from build123d import *

# Parameters (mm, degrees)
EXTRUDE_1_DEPTH        = 195
CUT_EXTRUDE_1_DEPTH    = 10
PATTERN_LINEAR_1_COUNT = 50
PATTERN_LINEAR_1_PITCH = 20


with BuildPart() as part:
    # 草图1 → 凸台-拉伸1 (new, symmetric)
    with BuildSketch(Plane.XY):
        with BuildLine():
            Line((0, 19.218912653), (1, 19.218912653))
            Line((1, 19.218912653), (1, 16.218912653))
            ThreePointArc((1, 16.218912653), (0.414213562, 14.80469909), (-1, 14.218912653))
            Line((-1, 14.218912653), (-4.5, 14.218912653))
            ThreePointArc((-4.5, 14.218912653), (-5.207106781, 13.926019434), (-5.5, 13.218912653))
            Line((-5.5, 13.218912653), (-5.5, -9.781087347))
            ThreePointArc((-5.5, -9.781087347), (-5.207106781, -10.488194128), (-4.5, -10.781087347))
            Line((-4.5, -10.781087347), (-1, -10.781087347))
            ThreePointArc((-1, -10.781087347), (0.414213562, -11.366873785), (1, -12.781087347))
            Line((1, -12.781087347), (1, -15.781087347))
            Line((1, -15.781087347), (0, -15.781087347))
            Line((0, -15.781087347), (0, -12.781087347))
            ThreePointArc((0, -12.781087347), (-0.292893219, -12.073980566), (-1, -11.781087347))
            Line((-1, -11.781087347), (-4.5, -11.781087347))
            ThreePointArc((-4.5, -11.781087347), (-5.914213562, -11.19530091), (-6.5, -9.781087347))
            Line((-6.5, -9.781087347), (-6.5, 13.218912653))
            ThreePointArc((-6.5, 13.218912653), (-5.914213562, 14.633126215), (-4.5, 15.218912653))
            Line((-4.5, 15.218912653), (-1, 15.218912653))
            ThreePointArc((-1, 15.218912653), (-0.292893219, 15.511805872), (0, 16.218912653))
            Line((0, 16.218912653), (0, 19.218912653))
        make_face()
    extrude(amount=EXTRUDE_1_DEPTH, both=True)

    # 草图2 → 切除-拉伸1 (cut)
    with BuildSketch(Plane(origin=(-5.5, 0, 0), x_dir=(0, 0, -1), z_dir=(1, 0, 0))):
        with BuildLine():
            Line((-183.75, 3.718912653), (-176.25, 3.718912653))
            ThreePointArc((-176.25, 3.718912653), (-174.25, 1.718912653), (-176.25, -0.281087347))
            Line((-176.25, -0.281087347), (-183.75, -0.281087347))
            ThreePointArc((-183.75, -0.281087347), (-185.75, 1.718912653), (-183.75, 3.718912653))
        make_face()
    cut_extrude_1 = extrude(amount=-CUT_EXTRUDE_1_DEPTH, mode=Mode.SUBTRACT)

    # 阵列(线性)1: 切除-拉伸1 ×50
    with Locations(*[(0, 0, -i * PATTERN_LINEAR_1_PITCH) for i in range(1, PATTERN_LINEAR_1_COUNT)]):
        add(cut_extrude_1, mode=Mode.SUBTRACT)


solid = part.part
Input: part model. Units: mm. Frame: model coordinates. Give positions to 0.01 mm unless a question says otherwise; leave off trailing zeros. Order: outer loops, then holes, each group sorted by start corner. A loop starts at its lowest first (then second) coordinate and runs counter-clockwise, first axis right, second up. Notation, with made-up numbers: M 40.25,64.5 L 97.25,64.5 A27 cw 97.25,83.5 Z; hole C -34,-20 d2. An arc over 180 degrees is marked long. Answer as a JSON object with one key per item and string values.
1. Cut plane A-A, the plane x = -3. Output: boundary loops of the cut face in (y, z), and give its area (3 significant figures).
Result sheet:
{"outline": "M -11.78,-195 L -10.78,-195 L -10.78,195 L -11.78,195 Z; M 14.22,-195 L 15.22,-195 L 15.22,195 L 14.22,195 Z", "area": "780 mm²"}
2. Pull-direction query (Y, two-part tool) for faces 1 (the flat face through (-6, -8, -195)), 2 (the flat face through (-5.5, -1, 3)); classes: +Y half, -Y half, draft (parallel to the pull), parting line (faces both ways), or undercut.
Result sheet:
{"face 1": "draft", "face 2": "undercut"}
3. Cut plane B-B, the plane z = 111. Output: boundary loops of the cut face in (x, y), and give its area (3 significant figures).
Result sheet:
{"outline": "M -6.5,-9.78 A2 ccw -4.5,-11.78 L -1,-11.78 A1 cw 0,-12.78 L 0,-15.78 L 1,-15.78 L 1,-12.78 A2 ccw -1,-10.78 L -4.5,-10.78 A1 cw -5.5,-9.78 L -5.5,13.22 A1 cw -4.5,14.22 L -1,14.22 A2 ccw 1,16.22 L 1,19.22 L 0,19.22 L 0,16.22 A1 cw -1,15.22 L -4.5,15.22 A2 ccw -6.5,13.22 Z", "area": "45.4 mm²"}
4. First-contact query: P1, Ø1.5, axis at y = 3, z = 6, coming from the +X side; P2, Ø1.1, axis at x = -6, z = -180.5, coming from the -Y side; P3, Ø2.5, axis at y = -14.5, z = 84, coming from the -X side. Flat tips, straight axial feed; report the tip coordinate or a pass-through.
Result sheet:
{"P1": "x = -5.5", "P2": "y = -11.54", "P3": "x = 0"}
5. Ray query, line 1 (Y direction, x = -0.75, z = 29); line 2 (Y direction, x = -1.25, z = -68.5); line 3 (X direction, y = -4, z = -155.5). Return the intervals inside material, ascending. Write a range as [from, to].
Result sheet:
{"line 1": "[-11.81, -10.8], [14.23, 15.25]", "line 2": "[-11.78, -10.78], [14.22, 15.22]", "line 3": "[-6.5, -5.5]"}
